Work out the finished part from the listing and answer in its coordinate system (mm). A direction names the side the tool comes from. Round coordinates to 2 decimals unless told otherwise and drop trailing zeros. Order: outer loops, then holes, each group sorted by start corner. A loop starts at its lowest first (then second) coordinate and runs counter-clockwise, first axis right, second up. Notation, with made-up numbers: (43.5, 20.25) - (65.5, 20.25) arc R28 ccw to (65.5, 44.25) - close; hole circle Ø6 at (45, 32.5). An arc over 180 degrees is marked (long way). Use one line per item in the form item = value. Start each with the question number.
Q1. Given P1, Ø2, axis at x = 0, z = 15.65, coming from the +Y side; P2, Ø10, axis at y = 26.5, z = -15.5, coming from the +X side; P3, Ø9.5, axis at x = 0, z = 0, coming from the -Y side; P4, Ø8, axis at y = 3.5, z = -7, coming from the -X side, each flat-ended and moving along its own axis, determine where each tip first touches the part or whether it passes through.
Q2. Which of the six approach directions +Z, -Z, +X, -X, +Y, -Y give full straight-line access (tool end or side, diameter ignored) to faces 1 (the cylindrical face through (9.36, 26.3, 5.97)), 2 (the flat face through (-8, 30, 8)), 3 (the flat face through (5, 8, 0))?
Q3. Find the intervals of material crossed by line 1 (X direction, y = 28.25, z = 0); line 2 (X direction, y = 16.5, z = 0); line 3 (Y direction, x = 0.5, z = 5), in increasing order. Write a range as [from, to].
Q4. The part is cut by section C-C on y = 18. Determine the outline of the cut face in (x, z).
Q5. For a pull along Z with two mould halves and no side action, classify faces 4 (the flat face through (-8.4, 0, 8.4)), 5 (the cylindrical face through (1.262, 15.098, 4.006)), 6 (the cylindrical face through (-19.524, 14.797, -4.336)) as +Z half, -Z half, draft (parallel to the pull), parting line (faces both ways), or undercut.
Q6. The part is cut by section A-A on x = 0. State how many separate pieces and enclosed holes the cut face has, plus the area to 3 significant figures.
Q7. The part is cut by section D-D on y = 27.5. Determine the outline of the cut face in (x, z), plus the area to 3 significant figures.
from build123d import *

# Parameters (mm, degrees)
SKETCH2_R           = 20
BOSS_EXTRUDE1_DEPTH = 30
SKETCH3_R           = 11.1
CUT_EXTRUDE1_DEPTH  = 8
CUT_EXTRUDE2_START  = -8
SKETCH4_R           = 11.1
CUT_EXTRUDE2_DEPTH  = 8
SKETCH5_R           = 1.7
CUT_EXTRUDE3_DEPTH  = 42.231056256
SKETCH6_R           = 4.2
CUT_EXTRUDE4_DEPTH  = 36.832945734
FILLET1_R           = 0.5
FILLET2_R           = 0.5


with BuildPart() as part:
    # Sketch2 → Boss-Extrude1 (new body)
    with BuildSketch(Plane(origin=(0, 0, 0), x_dir=(1, 0, 0), z_dir=(0, 1, 0))):
        with Locations(Location((0, 0, 0), (0, 0, 270))):
            Circle(SKETCH2_R)
    extrude(amount=BOSS_EXTRUDE1_DEPTH)

    # Sketch3 → Cut-Extrude1 (cut)
    with BuildSketch(Plane(origin=(0, 30, 0), x_dir=(1, 0, 0), z_dir=(0, 1, 0))):
        with Locations(Location((0, 0, 0), (0, 0, 270))):
            Circle(SKETCH3_R)
    extrude(amount=-CUT_EXTRUDE1_DEPTH, mode=Mode.SUBTRACT)

    # Sketch4 → Cut-Extrude2 (cut)
    with BuildSketch(Plane(origin=(0, 0, 0), x_dir=(-1, 0, 0), z_dir=(0, -1, 0)).offset(CUT_EXTRUDE2_START)):
        with Locations(Location((0, 0, 0), (0, 0, 270))):
            Circle(SKETCH4_R)
    extrude(amount=CUT_EXTRUDE2_DEPTH, mode=Mode.SUBTRACT)

    # Sketch5 → Cut-Extrude3 (cut, through all)
    with BuildSketch(Plane(origin=(0, 30, 0), x_dir=(1, 0, 0), z_dir=(0, 1, 0))):
        with Locations(Location((0, 15.65, 0), (0, 0, 270))):
            Circle(SKETCH5_R)
        with Locations(Location((-15.65, 0, 0), (0, 0, 270))):
            Circle(SKETCH5_R)
        with Locations(Location((0, -15.65, 0), (0, 0, 270))):
            Circle(SKETCH5_R)
        with Locations(Location((15.65, 0, 0), (0, 0, 270))):
            Circle(SKETCH5_R)
    extrude(amount=-CUT_EXTRUDE3_DEPTH, mode=Mode.SUBTRACT)

    # Sketch6 → Cut-Extrude4 (cut, through all)
    with BuildSketch(Plane(origin=(0, 22, 0), x_dir=(1, 0, 0), z_dir=(0, 1, 0))):
        with Locations(Location((0, 0, 0), (0, 0, 270))):
            Circle(SKETCH6_R)
    extrude(amount=-CUT_EXTRUDE4_DEPTH, mode=Mode.SUBTRACT)

    # Fillet1
    fillet1_edges = [part.edges().sort_by_distance(p)[0] for p in [
        (0, 22, -11.1),
    ]]
    fillet(fillet1_edges, radius=FILLET1_R)

    # Fillet2
    fillet2_edges = [part.edges().sort_by_distance(p)[0] for p in [
        (0, 8, -11.1),
        (0, 0, -11.1),
        (0, 0, -20),
        (0, 30, -20),
    ]]
    fillet(fillet2_edges, radius=FILLET2_R)


solid = part.part
Found:
q1.P1 = through
q1.P2 = 17.02
q1.P3 = 8
q1.P4 = -19.77
q2.face_1 = +Y
q2.face_2 = +Z, -Z, +X, -X, +Y
q2.face_3 = -Y
q3.line_1 = [-20, -17.35], [-13.95, -11.1], [11.1, 13.95], [17.35, 20]
q3.line_2 = [-20, -17.35], [-13.95, -4.2], [4.2, 13.95], [17.35, 20]
q3.line_3 = [8, 22]
q4.outline = circle Ø40 at (0, 0); hole circle Ø3.4 at (-15.65, 0); hole circle Ø8.4 at (0, 0); hole circle Ø3.4 at (0, -15.65); hole circle Ø3.4 at (0, 15.65); hole circle Ø3.4 at (15.65, 0)
q5.face_4 = draft
q5.face_5 = undercut
q5.face_6 = parting line
q6.separate_pieces = 4
q6.enclosed_holes = 0
q6.area = 523 mm²
q7.outline = circle Ø40 at (0, 0); hole circle Ø3.4 at (-15.65, 0); hole circle Ø22.2 at (0, 0); hole circle Ø3.4 at (0, -15.65); hole circle Ø3.4 at (0, 15.65); hole circle Ø3.4 at (15.65, 0)
q7.area = 833 mm²
